Model file for the job. Use its own axes, mm. A direction names the side the tool comes from. Round coordinates to 2 decimals unless told otherwise and drop trailing zeros. Write each loop counter-clockwise with the first axis right and the second up, starting at its lowest first coordinate (ties: lowest second). Pieces come first, ordered by that corner, then holes.
```python
from build123d import *

# Parameters (mm, degrees)
SALIENTE_EXTRUIR1_DEPTH = 3
CROQUIS2_R              = 1.5
CORTAR_EXTRUIR1_DEPTH   = 4


with BuildPart() as part:
    # Croquis1 → Saliente-Extruir1 (new body)
    with BuildSketch(Plane.XY):
        with BuildLine():
            ThreePointArc((-10, -51.071091654), (0, -45.25), (10, -51.071091654))
            Line((10, -51.071091654), (10, 51.071091654))
            ThreePointArc((10, 51.071091654), (0, 45.25), (-10, 51.071091654))
            Line((-10, 51.071091654), (-10, -51.071091654))
        make_face()
        with BuildLine():
            ThreePointArc((-10, 51.071091654), (0, 45.25), (10, 51.071091654))
            Line((10, 51.071091654), (10, 56.75))
            Line((10, 56.75), (-10, 56.75))
            Line((-10, 56.75), (-10, 51.071091654))
        make_face()
        with BuildLine():
            Line((10, 56.75), (10, 51.071091654))
            ThreePointArc((10, 51.071091654), (11.118677979, 53.813164969), (11.5, 56.75))
            ThreePointArc((11.5, 56.75), (-2.936835031, 67.868677979), (-10, 51.071091654))
            Line((-10, 51.071091654), (-10, 56.75))
            Line((-10, 56.75), (10, 56.75))
        make_face()
        with BuildLine():
            Line((10, -51.071091654), (10, -56.75))
            Line((10, -56.75), (-10, -56.75))
            Line((-10, -56.75), (-10, -51.071091654))
            ThreePointArc((-10, -51.071091654), (-2.936835031, -67.868677979), (11.5, -56.75))
            ThreePointArc((11.5, -56.75), (11.118677979, -53.813164969), (10, -51.071091654))
        make_face()
        with BuildLine():
            Line((-10, -56.75), (10, -56.75))
            Line((10, -56.75), (10, -51.071091654))
            ThreePointArc((10, -51.071091654), (0, -45.25), (-10, -51.071091654))
            Line((-10, -51.071091654), (-10, -56.75))
        make_face()
    extrude(amount=SALIENTE_EXTRUIR1_DEPTH)

    # Croquis2 → Cortar-Extruir1 (cut, through all)
    with BuildSketch(Plane.XY.offset(3)):
        with Locations((0, 15)):
            Circle(CROQUIS2_R)
        with Locations((0, -15)):
            Circle(CROQUIS2_R)
        with Locations((0, 56.75)):
            Circle(CROQUIS2_R)
        with Locations((0, -56.75)):
            Circle(CROQUIS2_R)
    extrude(amount=-CORTAR_EXTRUIR1_DEPTH, mode=Mode.SUBTRACT)


solid = part.part
```
1) Flat gauge pins, fed straight in: pin 1 Ø6 at (x, y) = (-6, -14) entering from -Z; pin 2 Ø2.5 at (x, y) = (0, -15) entering from +Z. Where does each tip first touch, or does it go through?
2) Cut at A-A on y = 15. List the corners of the cut face in (x, z), and give its area (3 significant figures).
3) Cut at D-D on x = 7.75. List the corners of the cut face in (y, z), and give its area (3 significant figures).
4) Wall check: probe 1 along Y at (x, z) = (0, 0.75); probe 2 along Y at (x, z) = (-1, 2.75); probe 3 along X at (y, z) = (-36, 0.4). Give the ranges that are in metal, low to high.
5) Cut at B-B on z = 1.35. List the corners of the cut face in (x, y), and give its area (3 significant figures).
6) Which spindle directions (+Z, -Z, +X, -X, +Y, -Y) get a long thin tool onto all of the face, cutting with end or side? Do faces 5 (the face through (-0.325, -16.464, 1.521)), 6 (the face through (-10, 1, 1)). Say none if no direction does.
7) Cut at C-C on x = 0. List the corners of the cut face in (y, z), and give its area (4 significant figures).
8) Pull direction X, two halves, no side cores. Call faces 1 (the face through (-0.195, 58.237, 1.521)), 2 (the face through (10, -1, 1)), 3 (the face through (-0.195, -55.263, 1.521)), 4 (the face through (0, 1, 3)): released by +X, released by -X, zero draft, split by the parting line, or undercut.
Result sheet:
1. pin 1: stops at z = 0
1. pin 2: passes through
2. outline: (-10, 0) - (-1.5, 0) - (-1.5, 3) - (-10, 3) - close; (1.5, 0) - (10, 0) - (10, 3) - (1.5, 3) - close
2. area: 51.0 mm2
3. outline: (-65.25, 0) - (65.25, 0) - (65.25, 3) - (-65.25, 3) - close
3. area: 391 mm2
4. probe 1: y = -68.25 to -58.25, -55.25 to -16.5, -13.5 to 13.5, 16.5 to 55.25, 58.25 to 68.25
4. probe 2: y = -68.21 to -57.87, -55.63 to -16.12, -13.88 to 13.88, 16.12 to 55.63, 57.87 to 68.21
4. probe 3: x = -10 to 10
5. outline: (-10, -51.07) arc R11.5 ccw (long way) to (10, -51.07) - (10, 51.07) arc R11.5 ccw (long way) to (-10, 51.07) - close; hole circle Ø3 at (0, -56.75); hole circle Ø3 at (0, -15); hole circle Ø3 at (0, 15); hole circle Ø3 at (0, 56.75)
5. area: 2,680 mm2
6. face 5: +Z, -Z
6. face 6: +Z, -Z, -X
7. outline: (-68.25, 0) - (-58.25, 0) - (-58.25, 3) - (-68.25, 3) - close; (-55.25, 0) - (-16.5, 0) - (-16.5, 3) - (-55.25, 3) - close; (-13.5, 0) - (13.5, 0) - (13.5, 3) - (-13.5, 3) - close; (16.5, 0) - (55.25, 0) - (55.25, 3) - (16.5, 3) - close; (58.25, 0) - (68.25, 0) - (68.25, 3) - (58.25, 3) - close
7. area: 373.5 mm2
8. face 1: undercut
8. face 2: released by +X
8. face 3: undercut
8. face 4: zero draft
